Check sheet for the modelled part. Datum: model origin and axes. Units: mm. Give positions to 0.01 mm unless a question says otherwise; leave off trailing zeros. Order: outer loops, then holes, each group sorted by start corner. A loop starts at its lowest first (then second) coordinate and runs counter-clockwise, first axis right, second up.
Item 1: Sectioned sample at C-C on y = -9. Record the boundary of the cut face in (x, z), and give its area (3 significant figures).
Item 2: Material ranges on line 1 along Y through (x, z) = (0, 1.6); line 2 along X through (y, z) = (-3.25, 3.3); line 3 along X through (y, z) = (-3.75, 0.9), recorded low to high.
Item 3: Gauge pin test, flat end, axial feed: P1, Ø3, axis at y = -1, z = 2, coming from the -X side. Record the tip position at first contact, or that the pin passes through.
Item 4: Sectioned sample at B-B on z = 3.3. Record the boundary of the cut face in (x, y).
Item 5: Sectioned sample at A-A on y = -5. Record the boundary of the cut face in (x, z).
Item 6: Release check for a two-part mould opening along Y. For faces 1 (the cylindrical face through (105, -5, 2)), 2 (the cylindrical face through (0, -7, 3)), 3 (the flat face through (49, 0, 2)), 4 (the flat face through (51, -5, 5)) record: released by +Y, released by -Y, zero draft, split by the parting line, or undercut.
from build123d import *

# Parameters (mm, degrees)
SKETCH1_W           = 100
SKETCH1_H           = 10
BOSS_EXTRUDE1_DEPTH = 5
SKETCH2_R           = 2
CUT_EXTRUDE1_DEPTH  = 106.59356041


with BuildPart() as part:
    # Sketch1 → Boss-Extrude1 (new body)
    with BuildSketch(Plane.XY):
        with BuildLine():
            Line((0, 0), (0, -10))
            ThreePointArc((0, -10), (-5, -5), (0, 0))
        make_face()
        with Locations((50, -5)):
            Rectangle(SKETCH1_W, SKETCH1_H)
        with BuildLine():
            ThreePointArc((100, 0), (105, -5), (100, -10))
            Line((100, -10), (100, 0))
        make_face()
    extrude(amount=BOSS_EXTRUDE1_DEPTH)

    # Sketch2 → Cut-Extrude1 (cut, through all)
    with BuildSketch(Plane.XY.offset(5)):
        with Locations((0, -5)):
            Circle(SKETCH2_R)
    extrude(amount=-CUT_EXTRUDE1_DEPTH, mode=Mode.SUBTRACT)


solid = part.part
Report:
1. outline: (-3, 0) - (103, 0) - (103, 5) - (-3, 5) - close
1. area: 530 mm2
2. line 1: y = -10 to -7, -3 to 0
2. line 2: x = -4.68 to -0.97, 0.97 to 104.68
2. line 3: x = -4.84 to -1.56, 1.56 to 104.84
3. P1: stops at x = -4.33
4. outline: (0, -10) - (100, -10) arc R5 ccw to (100, 0) - (0, 0) arc R5 ccw to start; hole circle Ø4 at (0, -5)
5. outline: (-5, 0) - (-2, 0) - (-2, 5) - (-5, 5) - close; (2, 0) - (105, 0) - (105, 5) - (2, 5) - close
6. face 1: split by the parting line
6. face 2: undercut
6. face 3: released by +Y
6. face 4: zero draft
